The model under review builds one solid part; all positions refer to its coordinate system, in mm. A direction names the side the tool comes from. Coordinates: 2 decimals unless noted, no trailing zeros. Order: outer loops, then holes, each group sorted by start corner. A loop starts at its lowest first (then second) coordinate and runs counter-clockwise, first axis right, second up. Notation, with made-up numbers: M 43,22.25 L 52,22.25 A23 cw 52,49.25 Z; hole C 41.25,85.5 d9. An arc over 180 degrees is marked long. Answer in a Markdown table with one row per item.
from build123d import *

# Parameters (mm, degrees)
BOSS_EXTRUDE1_DEPTH = 53.1
BOSS_EXTRUDE2_DEPTH = 6
SKETCH3_W           = 0.955506131
SKETCH3_H           = 0.5
BOSS_EXTRUDE3_DEPTH = 5
BOSS_EXTRUDE4_DEPTH = 6


with BuildPart() as part:
    # Sketch1 → Boss-Extrude1 (new body)
    with BuildSketch(Plane(origin=(0, 0, 0), x_dir=(0, 0, -1), z_dir=(1, 0, 0))):
        Polygon((0, 0), (12.5, 0), (12.5, 3.577441077), (3.577441077, 3.577441077), (3.577441077, 12.5), (0, 12.5), align=None)
    extrude(amount=BOSS_EXTRUDE1_DEPTH)

    # Sketch2 → Boss-Extrude2 (add)
    with BuildSketch(Plane.XY):
        with BuildLine():
            Line((9.4328, 10.2), (43.6672, 10.2))
            ThreePointArc((43.6672, 10.2), (45.262717366, 9.455998033), (45.718357588, 7.755525576))
            Line((45.718357588, 7.755525576), (45.059882111, 4.021125576))
            ThreePointArc((45.059882111, 4.021125576), (44.347522557, 2.787282634), (43.008724523, 2.3))
            Line((43.008724523, 2.3), (10.091275477, 2.3))
            ThreePointArc((10.091275477, 2.3), (8.752477443, 2.787282634), (8.040117889, 4.021125576))
            Line((8.040117889, 4.021125576), (7.381642412, 7.755525576))
            ThreePointArc((7.381642412, 7.755525576), (7.837282634, 9.455998033), (9.4328, 10.2))
        make_face()
    extrude(amount=BOSS_EXTRUDE2_DEPTH)

    # Sketch3 → Boss-Extrude3 (add)
    with BuildSketch(Plane.XZ):
        with Locations((1.917753066, -9.5)):
            Rectangle(SKETCH3_W, SKETCH3_H)
        with Locations((4.142246935, -9.5)):
            Rectangle(SKETCH3_W, SKETCH3_H)
        with Locations((48.957753066, -9.5)):
            Rectangle(SKETCH3_W, SKETCH3_H)
        with Locations((51.182246935, -9.5)):
            Rectangle(SKETCH3_W, SKETCH3_H)
    extrude(amount=BOSS_EXTRUDE3_DEPTH)

    # Sketch4 → Boss-Extrude4 (add)
    with BuildSketch(Plane.XY):
        Polygon((4.177995884, 4.261612802), (5.325991768, 6.25), (4.177995884, 8.238387198), (1.882004116, 8.238387198), (0.734008232, 6.25), (1.882004116, 4.261612802), align=None)
        Polygon((51.217995884, 4.261612802), (52.365991768, 6.25), (51.217995884, 8.238387198), (48.922004116, 8.238387198), (47.774008232, 6.25), (48.922004116, 4.261612802), align=None)
    extrude(amount=BOSS_EXTRUDE4_DEPTH)


solid = part.part
(1) Insertion check: P1, Ø6, axis at x = 11, z = 0, coming from the -Y side; P2, Ø1.1, axis at x = 49.5, z = 3, coming from the +Y side; P3, Ø2.5, axis at x = 3, z = 4, coming from the -Y side; P4, Ø3, axis at y = 7, z = -6.5, coming from the +X side. Each pin has a flat end and moves straight along its axis. Give the tip position at first contact, or say it passes through.
Report:
| item | result |
|---|---|
| P1 | y = 0 |
| P2 | y = 8.24 |
| P3 | y = 4.26 |
| P4 | through |
(2) Machinability: for faces 4 (the flat face through (26, 8, -3.577)), 5 (the flat face through (26, 10.2, 3)), 6 (the flat face through (3, 4.262, 3)), 7 (the flat face through (51, -2, -9.25)), which of the approach directions +Z, -Z, +X, -X, +Y, -Y give a long, thin tool a straight path to every point of the face, cutting with its end or side? Answer none if there is none.
Report:
| item | result |
|---|---|
| face 4 | -Z, +X, -X, +Y |
| face 5 | +Z, +X, -X, +Y |
| face 6 | +Z, -X, -Y |
| face 7 | +Z, +X, -X, -Y |
(3) Take a section at D-D (y = 8.75). Write out the cut boundary in (x, z).
Report:
| item | result |
|---|---|
| outline | M 0,-3.58 L 53.1,-3.58 L 53.1,0 L 45.65,0 L 45.65,6 L 7.45,6 L 7.45,0 L 0,0 Z |
(4) Take a section at C-C (x = 16). Write out the cut boundary in (y, z).
Report:
| item | result |
|---|---|
| outline | M 0,-12.5 L 3.58,-12.5 L 3.58,-3.58 L 12.5,-3.58 L 12.5,0 L 10.2,0 L 10.2,6 L 2.3,6 L 2.3,0 L 0,0 Z |
(5) Take a section at B-B (z = 1.25). Write out the cut boundary in (x, y), then the cut area to 3 significant figures.
Report:
| item | result |
|---|---|
| outline | M 0.73,6.25 L 1.88,4.26 L 4.18,4.26 L 5.33,6.25 L 4.18,8.24 L 1.88,8.24 Z; M 7.38,7.76 L 8.04,4.02 A2.08 ccw 10.09,2.3 L 43.01,2.3 A2.08 ccw 45.06,4.02 L 45.72,7.76 A2.08 ccw 43.67,10.2 L 9.43,10.2 A2.08 ccw Z; M 47.77,6.25 L 48.92,4.26 L 51.22,4.26 L 52.37,6.25 L 51.22,8.24 L 48.92,8.24 Z |
| area | 322 mm^2 |
(6) Take a section at A-A (y = -1.25). Write out the cut boundary in (x, z), then the cut area to 3 significant figures.
Report:
| item | result |
|---|---|
| outline | M 1.44,-9.75 L 2.4,-9.75 L 2.4,-9.25 L 1.44,-9.25 Z; M 3.66,-9.75 L 4.62,-9.75 L 4.62,-9.25 L 3.66,-9.25 Z; M 48.48,-9.75 L 49.44,-9.75 L 49.44,-9.25 L 48.48,-9.25 Z; M 50.7,-9.75 L 51.66,-9.75 L 51.66,-9.25 L 50.7,-9.25 Z |
| area | 1.91 mm^2 |
(7) To check wall thickness, follow line 1 (X direction, y = 6, z = 1); line 2 (Z direction, x = 23, y = 6.75); line 3 (Y direction, x = 22.5, z = -0.25). State the ranges of each line that lie inside material, in increasing order. Write a range as [from, to].
Report:
| item | result |
|---|---|
| line 1 | [0.88, 5.18], [7.69, 45.41], [47.92, 52.22] |
| line 2 | [-3.58, 6] |
| line 3 | [0, 12.5] |
(8) The part is to be moulded in two halves that separate along X. For faces 1 (the flat face through (1.3, 5.27, 2.96)), 2 (the flat face through (48.356, 7.258, 2.958)), 3 (the flat face through (26, 3.577, -8)), say which applies: +X half, -X half, draft (parallel to the pull), parting line (faces both ways), or undercut.
Report:
| item | result |
|---|---|
| face 1 | -X half |
| face 2 | undercut |
| face 3 | draft |
